Input: part model. Units: mm. Frame: model coordinates. Face numbers are marked on the shaded views. A direction names the side the tool comes from. Round coordinates to 2 decimals unless told otherwise and drop trailing zeros. Write each loop counter-clockwise with the first axis right and the second up, starting at its lowest first coordinate (ties: lowest second). Pieces come first, ordered by that corner, then holes. Notation, with made-up numbers: (-21, 38) - (-6, 38) arc R9 ccw to (-6, 49) - close; hole circle Ø1 at (88.25, -2). An arc over 180 degrees is marked (long way). Use one line per item in the form item = value.
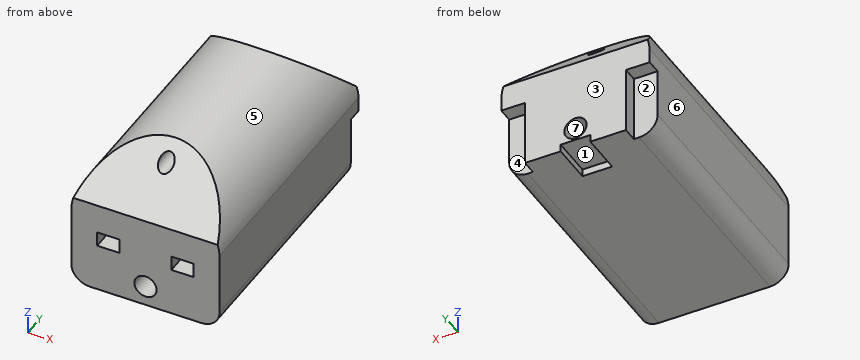
Autodesk Inventor part; units mm, degrees
ref_plane "Work Plane1" through (-10, 35, -20) normal (-1, 0, 0) x (0, -1, 0)
ref_plane "Work Plane2" through (0, 2, -2) normal (1, 0, 0) x (0, 0, -1)
ref_plane "Work Plane3" through (-20, 17.5, -9) normal (0, 1, 0) x (-1, 0, 0)
sketch "Sketch1" plane through (0, 0, 0) normal (0, 1, 0) x (-1, 0, 0)
  line L0 (0, 0) -> (20, 0)
  line L1 (20, 0) -> (20, -20)
  line L2 (20, -20) -> (0, -20)
  line L3 (0, -20) -> (0, 0)
  dimension "d0" = 20
  dimension "d1" = 20
extrude "Extrusion1" add sketch "Sketch1" along normal blind 35
sketch "Sketch3" plane through (0, 0, 0) normal (1, 0, 0) x (0, 0, -1)
  line L0 (0, 35) -> (20, 35)
  line L1 (20, 35) -> (0, 35)
  line L2 (20, 35) -> (12.5, 35)
  line L3 (12.5, 35) -> (14, 35)
  line L4 (12.5, 35) -> (11, 35)
  line L5 (14, 35) -> (18.5, 35)
  line L6 (18.5, 35) -> (18.5, 33)
  line L7 (18.5, 33) -> (14, 35)
  line L8 (11, 35) -> (6.5, 35)
  line L9 (6.5, 35) -> (6.5, 33)
  line L10 (6.5, 33) -> (11, 35)
  line L11 (6.5, 33) -> (18.5, 33)
  line L12 (11, 35) -> (11, 33)
  line L13 (14, 35) -> (14, 33)
  point P0 (0, 0)
  dimension "d55" = 7.5
  dimension "d56" = 1.5
  dimension "d57" = 1.5
  dimension "d58" = 4.5
  dimension "d59" = 2
  dimension "d60" = 4.5
  dimension "d61" = 2
extrude "Extrusion3" cut sketch "Sketch3" against normal blind 3.2 contours L0 L13 L11 L12
sketch "Sketch9" plane through (0, 33, -14) normal (0, 0, 1) x (1, 0, 0)
  line L0 (0, 0) -> (-3.2, 0)
  line L1 (-3.2, 2) -> (0, 2)
  line L2 (0, 0) -> (-3.2, 0)
  line L3 (-3.2, 0) -> (-3.2, 2)
  line L4 (-3.2, 2) -> (0, 2)
  line L5 (0, 2) -> (0, 0)
  point P0 (0, -33)
extrude "Extrusion9" cut sketch "Sketch9" against normal up to surface (6 mm away)
ref_plane "Work Plane1" through (-10, 35, -20) normal (-1, 0, 0) x (0, -1, 0)
sketch "Sketch4" plane through (0, 0, 0) normal (0, -1, 0) x (1, 0, 0)
  line L0 (-20, 0) -> (0, 0)
  line L1 (0, -20) -> (-20, -20)
  line L2 (0, -20) -> (-20, -20)
  line L3 (0, -20) -> (-3.5, -20)
  line L4 (-3.5, -20) -> (-3.5, -13.5)
  line L5 (-3.5, -13.5) -> (-3.5, -11.5)
  line L6 (-3.5, -11.5) -> (-6.5, -11.5)
  line L7 (-6.5, -11.5) -> (-6.5, -13.5)
  line L8 (-6.5, -13.5) -> (-3.5, -13.5)
  line L9 (-10, -20) -> (-10, 0)
  line L10 (-20, 0) -> (0, 0)
  line L11 (-16.5, -13.5) -> (-16.5, -11.5)
  line L12 (-16.5, -11.5) -> (-13.5, -11.5)
  line L13 (-13.5, -11.5) -> (-13.5, -13.5)
  line L14 (-13.5, -13.5) -> (-16.5, -13.5)
  dimension "d62" = 3.5
  dimension "d63" = 6.5
  dimension "d64" = 2
  dimension "d65" = 3
  dimension "d66" = 2
extrude "Extrusion4" cut sketch "Sketch4" against normal blind 2.5
fillet "Fillet3" radius 2.5 4 edges at (0, 17.5, 0) (-20, 17.5, 0) (-20, 17.5, -20) (0, 16.5, -20)
sketch "Sketch6" plane through (0, 35, 0) normal (0, 1, 0) x (1, 0, 0)
  line L0 (-2, 0) -> (-18, 0)
  line L1 (-10, 0) -> (-10, 20)
  line L2 (-18, 20) -> (-2, 20)
  line L3 (-10, 0) -> (-10, 1.25)
  circle A0 centre (-10, 10) radius 8.75
  line L4 (-10, 1.25) -> (-11, 1.25)
  line L5 (-10, 1.25) -> (-9, 1.25)
  line L6 (-10, 1.25) -> (-9, 1.25) construction
  line L7 (-9, 1.25) -> (-9, 20)
  line L8 (-2, 20) -> (-18, 20)
  line L9 (-9, 20) -> (-11, 20)
  line L10 (-11, 20) -> (-11, 1.25)
  circle A1 centre (-10, 17.25) radius 1.5
  circle A2 centre (-10, 2.25) radius 1
  point P0 (0, 0)
  point P1 (-11, 18.6927)
  point P2 (-11, 1.3073)
  point P3 (-9, 1.3073)
  point P4 (-9, 18.6927)
  dimension "d40" = 1.25
  dimension "d41" = 1
  dimension "d42" = 1
  dimension "d43" = 0
  dimension "d44" = 90
  dimension "d45" = 2
  dimension "d69" = 3
  dimension "d70" = 2
  dimension "d71" = 0
  dimension "d72" = 0
  dimension "d73" = 0
ref_plane "Work Plane2" through (0, 2, -2) normal (1, 0, 0) x (0, 0, -1)
sketch "Sketch7" plane through (0, 2, -2) normal (1, 0, 0) x (0, 0, -1)
  line L0 (-2, -2) -> (-2, 5.5)
  line L1 (-2, -2) -> (-2, 33)
  line L2 (-2, 5.5) -> (5.5, -2)
  line L3 (5.5, -2) -> (-2, -2)
  line L4 (7, -2) -> (7, 0.2)
  point P0 (-2, 0)
  point P1 (-2, 31)
  dimension "d36" = 7.5
  dimension "d37" = 45
extrude "Extrusion6" cut sketch "Sketch7" against normal up to surface (20 mm away)
extrude "Extrusion7" cut sketch "Sketch6" against normal up to surface (35 mm away) contours A2 L1 | L1 A2 | A1 L10 L1 | L1 A1 L7 | L7 A1 | A1 L10
sketch "Sketch8" plane through (0, 35, 0) normal (0, 1, 0) x (1, 0, 0)
  line L0 (-9, 18.6927) -> (-9, 1.3073)
  line L1 (-11, 1.3073) -> (-11, 18.6927)
  arc A0 (-11, 1.3073) -> (-9, 1.3073) centre (-10, 10) ccw
  arc A1 (-9, 18.6927) -> (-11, 18.6927) centre (-10, 10) ccw
  circle A2 centre (-10, 10) radius 8.75
  line L2 (-3.2, 11) -> (0, 11)
  line L3 (-20, 11) -> (-16.8, 11)
  line L4 (-16.8, 9) -> (-20, 9)
  line L5 (0, 9) -> (-3.2, 9)
  arc A3 (-20, 9) -> (0, 9) centre (-10, 10.0556) ccw
  line L6 (-3.2, 20) -> (-17.5, 20)
  arc A4 (-17.5, 20) -> (-20, 17.5) centre (-17.5, 17.5) ccw
  line L7 (-20, 17.5) -> (-20, 2.5)
  arc A5 (-20, 2.5) -> (-17.5, 0) centre (-17.5, 2.5) ccw
  line L8 (-17.5, 0) -> (-2.5, 0)
  arc A6 (-2.5, 0) -> (0, 2.5) centre (-2.5, 2.5) ccw
  line L9 (0, 2.5) -> (0, 11)
  line L10 (0, 11) -> (-3.2, 11)
  line L11 (-3.2, 11) -> (-3.2, 20)
  point P0 (0, 0)
  point P1 (-10, 0)
  dimension "d51" = 17.5
extrude "Extrusion8" cut sketch "Sketch8" against normal up to surface (35 mm away) contours L9 A6 L8 A3 | A3 L8 A5 L7
mirror "Mirror2" about plane through (-10, 35, -20) normal (-1, 0, 0) of "Extrusion3", "Extrusion9"
ref_plane "Work Plane3" through (-20, 17.5, -9) normal (0, 1, 0) x (-1, 0, 0)
mirror "Mirror3" about plane through (-20, 17.5, -9) normal (0, 1, 0) of "Extrusion6"
sketch "Sketch11" plane through (-3.2, 33, -20) normal (0, 0, -1) x (-1, 0, 0)
  line L0 (0, 2) -> (13.6, 2)
  line L1 (5.3, 2) -> (8.3, 2)
  line L2 (6.8, 2) -> (12.3, 2) construction
  line L3 (8.8, 2) -> (4.8, 2)
  line L4 (4.8, 2) -> (4.8, -3.5)
  line L5 (4.8, -3.5) -> (8.8, -3.5)
  line L6 (8.8, -3.5) -> (8.8, 2)
  point P0 (-3.2, -33)
  point P1 (6.8, 2)
  point P2 (6.8, 2)
  point P3 (4.8, 2)
  dimension "d76" = 4
  dimension "d77" = 5.5
  dimension "d78" = 0
  dimension "d79" = 0
extrude "Extrusion10" cut sketch "Sketch11" against normal blind 1
properties part number "BaseKnuckle"
(1) Cut plane C-C on z = -12. Output: boundary loops of the cut face in (x, y), then the cut area to 3 significant figures.
Derived:
outline = (-20, 0) - (-16.5, 0) - (-16.5, 2.5) - (-13.5, 2.5) - (-13.5, 0) - (-6.5, 0) - (-6.5, 2.5) - (-3.5, 2.5) - (-3.5, 0) - (0, 0) - (0, 33) - (-3.2, 33) - (-3.2, 35) - (-16.8, 35) - (-16.8, 33) - (-20, 33) - close
area = 672 mm^2
(2) Cut plane B-B on y = 13. Output: boundary loops of the cut face in (x, z), then the cut area to 3 significant figures.
Derived:
outline = (-20, -17.5) arc R2.5 ccw to (-17.5, -20) - (-2.5, -20) arc R2.5 ccw to (0, -17.5) - (0, -9) arc R10.06 ccw to (-20, -9) - close; hole circle Ø3 at (-10, -17.25); hole circle Ø2 at (-10, -2.25)
area = 345 mm^2
(3) First-contact query: pin 1 Ø3 at (x, z) = (-10, -2.25) entering from -Y; pin 2 Ø1.6 at (x, z) = (-19, -13.5) entering from +Y; pin 3 Ø1.2 at (x, y) = (-4.5, 1.5) entering from +Z. Flat tips, straight axial feed; report the tip coordinate or a pass-through.
Derived:
pin_1 = 3.75
pin_2 = 33
pin_3 = -5.4
(4) Access query for the marked faces 1, 2 and 3. Directions: +Z, -Z, +X, -X, +Y, -Y. A direction counts if a zero-diameter tool reaches every point of the face in a straight line with its end or side. Return the directions, or none.
Derived:
face_1 = -Z, +Y
face_2 = -Z, -X, +Y
face_3 = +Z, -Z, +X, -X, +Y
(5) Material intervals for L1, parallel to Z at x = -10, y = 13.5; L2, parallel to X at y = 16, z = -17.25; L3, parallel to Z at x = -5, y = 5, sorted ascending.
Derived:
L1 = -20 to -18.75, -15.75 to -3.25, -1.25 to 0
L2 = -20 to -11.5, -8.5 to 0
L3 = -20 to -2.5
(6) Draft query along X for the marked faces 4, 5, 6 and 7. Return one class per face: released by +X, released by -X, zero draft, split by the parting line, or undercut.
Derived:
face_4 = zero draft
face_5 = split by the parting line
face_6 = released by -X
face_7 = undercut
(7) Cut plane A-A on x = -10. Output: boundary loops of the cut face in (y, z), then the cut area to 3 significant figures.
Derived:
outline = (0, -20) - (29.5, -20) - (29.5, -19) - (35, -19) - (35, -18.75) - (0, -18.75) - close; (0, -15.75) - (35, -15.75) - (35, -7.5) - (30.75, -3.25) - (4.25, -3.25) - (0, -7.5) - close; (6.25, -1.25) - (28.75, -1.25) - (27.5, 0) - (7.5, 0) - close
area = 484 mm^2
(8) Cut plane D-D on z = -2.25. Output: boundary loops of the cut face in (x, y), then the cut area to 3 significant figures.
Derived:
outline = (-16.34, 5.25) - (-11, 5.25) - (-11, 29.75) - (-16.34, 29.75) - close; (-9, 5.25) - (-3.66, 5.25) - (-3.66, 29.75) - (-9, 29.75) - close
area = 262 mm^2
